The model under review builds one solid part; all positions refer to its coordinate system, in mm. A direction names the side the tool comes from. Round coordinates to 2 decimals unless told otherwise and drop trailing zeros. Write each loop counter-clockwise with the first axis right and the second up, starting at its lowest first coordinate (ties: lowest second). Pieces come first, ordered by that corner, then holes. Notation, with made-up numbers: (7.25, -9) - (20.25, -9) arc R32 cw to (20.25, 19) - close; hole circle Ø1 at (84.5, -30). An arc over 180 degrees is marked (long way). Return JSON: item names as keys, results as strings.
from build123d import *

# Parameters (mm, degrees)
BOSS_EXTRUDE1_DEPTH = 25.4
FILLET1_R           = 2.54
FILLET2_R           = 2.54
FILLET3_R           = 2.54
FILLET5_R           = 2.54
FILLET6_R           = 2.54


with BuildPart() as part:
    # Sketch1 → Boss-Extrude1 (new body)
    with BuildSketch(Plane.XY):
        Polygon((-12.7, 0), (12.7, 0), (13.550738686, -3.175), (19.900738686, -3.175), (19.900738686, -5.131589334), (11.971324019, -5.131589334), (11.14079156, -2.032), (-11.14079156, -2.032), (-11.991530246, -5.207), (-19.900738686, -5.207), (-19.900738686, -3.175), (-13.550738686, -3.175), align=None)
    extrude(amount=BOSS_EXTRUDE1_DEPTH)

    # Fillet1
    fillet1_edges = [part.edges().sort_by_distance(p)[0] for p in [
        (13.550738686, -3.175, 12.7),
    ]]
    fillet(fillet1_edges, radius=FILLET1_R)

    # Fillet2
    fillet2_edges = [part.edges().sort_by_distance(p)[0] for p in [
        (12.7, 0, 12.7),
    ]]
    fillet(fillet2_edges, radius=FILLET2_R)

    # Fillet3
    fillet3_edges = [part.edges().sort_by_distance(p)[0] for p in [
        (-11.991530246, -5.207, 12.7),
        (11.971324019, -5.131589334, 12.7),
    ]]
    fillet(fillet3_edges, radius=FILLET3_R)

    # Fillet5
    fillet5_edges = [part.edges().sort_by_distance(p)[0] for p in [
        (-13.550738686, -3.175, 12.7),
        (11.14079156, -2.032, 12.7),
        (-11.14079156, -2.032, 12.7),
    ]]
    fillet(fillet5_edges, radius=FILLET5_R)

    # Fillet6
    fillet6_edges = [part.edges().sort_by_distance(p)[0] for p in [
        (-12.7, 0, 12.7),
    ]]
    fillet(fillet6_edges, radius=FILLET6_R)


solid = part.part
(1) Wall thickness on line 1 (Y direction, x = -5.5, z = 11.75); line 2 (Y direction, x = 17.5, z = 23) (3 decimals); line 3 (X direction, y = -4.45, z = 14.75): over which ranges is each line inside the solid? List them lowest first.
Filled in:
{"line 1": "y = -2.03 to 0", "line 2": "y = -5.132 to -3.175", "line 3": "x = -19.9 to -12.13, 12.19 to 19.9"}
(2) Clearance check with flat-ended pins moving along their axes: pin 1 Ø3.5 at (x, z) = (17.5, 16) entering from +Y (3 decimals); pin 2 Ø6.5 at (x, z) = (17.5, 18.5) entering from -Y; pin 3 Ø9 at (x, z) = (4, 7.5) entering from -Y. State where each tip first meets the part, or that it passes through.
Filled in:
{"pin 1": "stops at y = -3.175", "pin 2": "stops at y = -5.13", "pin 3": "stops at y = -2.03"}
(3) Add section B-B (x = 15). Write out the cut boundary in (y, z), plus the area to 3 significant figures.
Filled in:
{"outline": "(-5.13, 0) - (-3.13, 0) - (-3.13, 25.4) - (-5.13, 25.4) - close", "area": "51.0 mm2"}
(4) Mouldability with a two-part tool opening along X and no side actions: class faces 1 (the cylindrical face through (12.535, -4.72, 12.878)), 2 (the flat face through (19.901, -4, 13)), 3 (the flat face through (-18, -3.175, 13)) as released by +X, released by -X, zero draft, split by the parting line, or undercut.
Filled in:
{"face 1": "undercut", "face 2": "released by +X", "face 3": "zero draft"}
(5) For faces 4 (the flat face through (18, -3.175, 13)), 5 (the flat face through (0, -1, 0)), 6 (the flat face through (17, -5.132, 13)), 7 (the cylindrical face through (-14.062, -2.729, 12.878)), 8 (the flat face through (0, -2.032, 13)), list the 3-axis set-ups (+Z, -Z, +X, -X, +Y, -Y) from which the entire face can be reached by the end or side of a thin tool; tool diameter is ignored.
Filled in:
{"face 4": "+Z, -Z, +X, +Y", "face 5": "-Z, +X, -X, +Y, -Y", "face 6": "+Z, -Z, +X, -Y", "face 7": "+Z, -Z, -X, +Y", "face 8": "+Z, -Z, -Y"}
(6) Add section A-A (x = 4.5). Write out the cut boundary in (y, z), plus the area to 3 significant figures.
Filled in:
{"outline": "(-2.03, 0) - (0, 0) - (0, 25.4) - (-2.03, 25.4) - close", "area": "51.6 mm2"}
